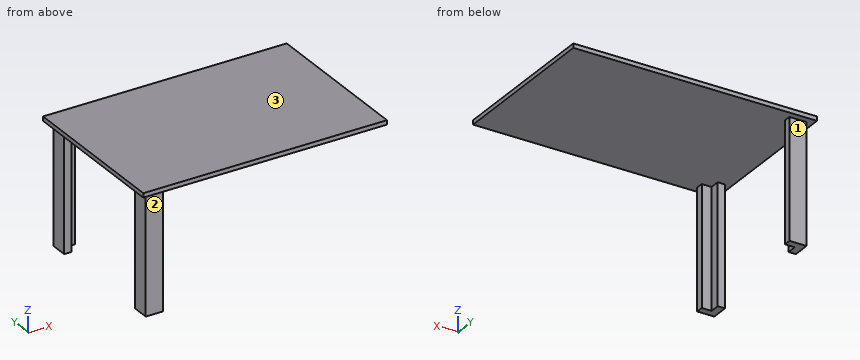
```python
from build123d import *

# Parameters (mm, degrees)
F1_DEPTH = 736.6
F0_W     = 1447.8
F0_H     = 952.5
F3_DEPTH = 25.4


with BuildPart() as f1:
    # F0 (on Top) → F1 (new body)
    with BuildSketch(Plane.XY):
        Polygon((-1308.1, 438.15), (-1409.7, 438.15), (-1409.7, 336.55), (-1366.275751, 336.55), (-1366.275751, 394.725751), (-1308.1, 394.725751), align=None)
    extrude(amount=-F1_DEPTH)



with BuildPart() as f2_1:
    # F2: instance of F1
    add(f1.part.mirror(Plane.XZ))


with BuildPart() as f1_1:
    add(f1.part)

    add(f2_1.part)  # F3 merges F2_1
    # F0 (on Top) → F3 (join)
    with BuildSketch(Plane.XY):
        with Locations((-723.9, 0)):
            Rectangle(F0_W, F0_H)
        Polygon((-1409.7, 336.55), (-1409.7, 438.15), (-1308.1, 438.15), (-1308.1, 394.725751), (-1366.275751, 394.725751), (-1366.275751, 336.55), align=None, mode=Mode.SUBTRACT)
    extrude(amount=-F3_DEPTH)


solid = f1_1.part
```
Can you work these out from the model? Positions are in its coordinate system, mm. Face numbers are marked on the shaded views. A direction names the side the tool comes from. Coordinates: 2 decimals unless noted, no trailing zeros. Loops run counter-clockwise (first coordinate to the right, second up) from the corner with the lowest first, then second, coordinate; pieces in that order, holes last.
1) Imagine slicing it at D-D on x = -299. List the corners of the cut face in (y, z) for me, plus the area to 3 significant figures.
2) Which directions (+Z, -Z, +X, -X, +Y, -Y) give clear straight access to the entire face, cutting with the end or side of a thin tool? Please do the marked faces 1, 2 and 3.
3) For pin 1 (1 mm diameter, centred on x = -864, y = 376.5, fed in from +Z); pin 2 (8 mm diameter, centred on x = -826, y = -352.5, fed in from -Z); pin 3 (13 mm diameter, centred on x = -1394, z = -492.5, fed in from -Y), each with a flat end and sliding along its axis, tell me the tip position at first contact or that it passes through.
4) Imagine slicing it at B-B on x = -1333.5. List the corners of the cut face in (y, z) for me.
5) Imagine slicing it at C-C on y = -127. List the corners of the cut face in (x, z) for me, plus the area to 3 significant figures.
6) Imagine slicing it at A-A on z = -645. List the corners of the cut face in (x, y) for me, plus the area to 3 significant figures.
7) I need wall thicknesses on probe 1 along Z at (x, y) = (-1127, 251); probe 2 along X at (y, z) = (-420.5, -121); probe 3 along X at (y, z) = (-363.5, -52.5). Which ranges of each line are inside material? Lowest first, please.
Completed:
1. outline: (-476.25, -25.4) - (476.25, -25.4) - (476.25, 0) - (-476.25, 0) - close
1. area: 24,200 mm2
2. face 1: -Z, +X, -X, +Y
2. face 2: -Z, +X, -X, -Y
2. face 3: +Z, +X, -X, +Y, -Y
3. pin 1: stops at z = 0
3. pin 2: stops at z = -25.4
3. pin 3: stops at y = -438.15
4. outline: (-476.25, -25.4) - (-438.15, -25.4) - (-438.15, -736.6) - (-394.73, -736.6) - (-394.73, -25.4) - (394.73, -25.4) - (394.73, -736.6) - (438.15, -736.6) - (438.15, -25.4) - (476.25, -25.4) - (476.25, 0) - (-476.25, 0) - close
5. outline: (-1447.8, -25.4) - (0, -25.4) - (0, 0) - (-1447.8, 0) - close
5. area: 36,800 mm2
6. outline: (-1409.7, -438.15) - (-1308.1, -438.15) - (-1308.1, -394.73) - (-1366.28, -394.73) - (-1366.28, -336.55) - (-1409.7, -336.55) - close; (-1409.7, 336.55) - (-1366.28, 336.55) - (-1366.28, 394.73) - (-1308.1, 394.73) - (-1308.1, 438.15) - (-1409.7, 438.15) - close
6. area: 13,900 mm2
7. probe 1: z = -25.4 to 0
7. probe 2: x = -1409.7 to -1308.1
7. probe 3: x = -1409.7 to -1366.28
